```python
from build123d import *

# Parameters (mm, degrees)
BOSS_EXTRUDE1_DEPTH = 6.35
FILLET1_R           = 3.302
FILLET2_R           = 3.302


with BuildPart() as part:
    # Sketch1 → Boss-Extrude1 (new body)
    with BuildSketch(Plane.XY):
        with BuildLine():
            Line((-43.182028134, 76.689298909), (-24.787442952, -5.544607461))
            ThreePointArc((-24.787442952, -5.544607461), (0, -25.4), (24.787442952, -5.544607461))
            Line((24.787442952, -5.544607461), (43.182028134, 76.689298909))
            ThreePointArc((43.182028134, 76.689298909), (0, 88.011), (-43.182028134, 76.689298909))
        make_face()
        with BuildLine():
            Line((-6.704060429, 15.0876), (6.704060429, 15.0876))
            ThreePointArc((6.704060429, 15.0876), (11.674332957, 11.674332957), (15.0876, 6.704060429))
            Line((15.0876, 6.704060429), (15.0876, -6.704060429))
            ThreePointArc((15.0876, -6.704060429), (11.674332957, -11.674332957), (6.704060429, -15.0876))
            Line((6.704060429, -15.0876), (-6.704060429, -15.0876))
            ThreePointArc((-6.704060429, -15.0876), (-11.674332957, -11.674332957), (-15.0876, -6.704060429))
            Line((-15.0876, -6.704060429), (-15.0876, 6.704060429))
            ThreePointArc((-15.0876, 6.704060429), (-11.674332957, 11.674332957), (-6.704060429, 15.0876))
        make_face(mode=Mode.SUBTRACT)
        with BuildLine():
            ThreePointArc((-34.124988821, 73.18127185), (0, 80.7466), (34.124988821, 73.18127185))
            ThreePointArc((34.124988821, 73.18127185), (35.218416261, 70.177102101), (32.214247077, 69.083673111))
            ThreePointArc((32.214247077, 69.083673111), (0, 76.2254), (-32.214247077, 69.083673111))
            ThreePointArc((-32.214247077, 69.083673111), (-35.218416261, 70.177102101), (-34.124988821, 73.18127185))
        make_face(mode=Mode.SUBTRACT)
    extrude(amount=BOSS_EXTRUDE1_DEPTH)

    # Fillet1
    fillet1_edges = [part.edges().sort_by_distance(p)[0] for p in [
        (-15.0876, 6.704060429, 3.175),
        (-15.0876, -6.704060429, 3.175),
        (-6.704060429, -15.0876, 3.175),
        (6.704060429, -15.0876, 3.175),
        (15.0876, -6.704060429, 3.175),
        (15.0876, 6.704060429, 3.175),
        (6.704060429, 15.0876, 3.175),
        (-6.704060429, 15.0876, 3.175),
    ]]
    fillet(fillet1_edges, radius=FILLET1_R)

    # Fillet2
    fillet2_edges = [part.edges().sort_by_distance(p)[0] for p in [
        (43.182028134, 76.689298909, 3.175),
        (-43.182028134, 76.689298909, 3.175),
    ]]
    fillet(fillet2_edges, radius=FILLET2_R)


solid = part.part
```
Model file for the job. Use its own axes, mm. A direction names the side the tool comes from. Coordinates: 2 decimals unless noted, no trailing zeros. Write each loop counter-clockwise with the first axis right and the second up, starting at its lowest first coordinate (ties: lowest second). Pieces come first, ordered by that corner, then holes. Notation, with made-up numbers: (-23, 14) - (-3, 14) arc R16 cw to (-3, 42) - close; hole circle Ø10 at (15, 73.25). An arc over 180 degrees is marked (long way). Use a Markdown table: item, result. Add a question column.
Item 1: Drop flat-ended pins along their axis: pin 1 (1.5 mm diameter, centred on y = -4.5, z = 1.5, fed in from -X); pin 2 (1 mm diameter, centred on x = -18, z = 5, fed in from +Y); pin 3 (1.5 mm diameter, centred on y = 43.5, z = 5, fed in from -X); pin 4 (12 mm diameter, centred on x = -32.5, y = 45, fed in from -Z). Give the stop position or say it passes through.
Item 2: Band-saw the part on B-B, the plane y = 79.5. Write the cut outline in (x, z), and give its area (3 significant figures).
Item 3: 3-axis set-ups, long thin cutter, end or side, ignore diameter. For faces 1 (the face through (-11.73, 11.62, 3.13)), 2 (the face through (-1, 45, 0)): which of +Z, -Z, +X, -X, +Y, -Y reach the whole face in a straight line?
Item 4: Drill centre lines: line 1 along Y through (x, z) = (0.5, 4.25); line 2 along Y through (x, z) = (3.5, 3.5) (3 decimals); line 3 along Y through (x, z) = (16.5, 1.5). Where is each one in solid material? Low to high.
Item 5: Band-saw the part on D-D, the plane y = -1.5. Write the cut outline in (x, z).
Item 6: Band-saw the part on A-A, the plane z = 3.5. Write the cut outline in (x, y).
Item 7: Two-plate mould, pull along X, no slides. Class faces 3 (the face through (42.4, 76.39, 3.22)), 4 (the face through (-42.425, 76.339, 3.219)), 5 (the face through (0, -15.088, 3)), 6 (the face through (0.6, 88.01, 3.13)): pulls with the +X half, pulls with the -X half, needs draft (parallel to the pull), parting line crosses it, or undercut.
Item 8: Band-saw the part on C-C, the plane x = -4. Write the cut outline in (y, z), and give its area (3 significant figures).
A:
| question | item | result |
|---|---|---|
| 1 | pin 1 | stops at x = -25.19 |
| 1 | pin 2 | stops at y = 86.25 |
| 1 | pin 3 | stops at x = -35.93 |
| 1 | pin 4 | stops at z = 0 |
| 2 | outline | (-37.76, 0) - (-14.13, 0) - (-14.13, 6.35) - (-37.76, 6.35) - close; (14.13, 0) - (37.76, 0) - (37.76, 6.35) - (14.13, 6.35) - close |
| 2 | area | 300 mm² |
| 3 | face 1 | +Z, -Z |
| 3 | face 2 | -Z, +X, -X, +Y, -Y |
| 4 | line 1 | y = -25.4 to -15.09, 15.09 to 76.22, 80.75 to 88.01 |
| 4 | line 2 | y = -25.158 to -15.088, 15.088 to 76.145, 80.671 to 87.941 |
| 4 | line 3 | y = -19.31 to 74.42, 79.04 to 86.45 |
| 5 | outline | (-25.69, 0) - (-15.09, 0) - (-15.09, 6.35) - (-25.69, 6.35) - close; (15.09, 0) - (25.69, 0) - (25.69, 6.35) - (15.09, 6.35) - close |
| 6 | outline | (-42.64, 74.26) - (-24.79, -5.54) arc R25.4 ccw to (24.79, -5.54) - (42.64, 74.26) arc R3.3 ccw to (40.95, 77.9) arc R88.01 ccw to (-40.95, 77.9) arc R3.3 ccw to start; hole (-34.12, 73.18) arc R2.26 ccw to (-32.21, 69.08) arc R76.23 cw to (32.21, 69.08) arc R2.26 ccw to (34.12, 73.18) arc R80.75 ccw to start; hole (-15.09, -5.96) arc R3.3 ccw to (-14.73, -7.45) arc R16.51 ccw to (-7.45, -14.73) arc R3.3 ccw to (-5.96, -15.09) - (5.96, -15.09) arc R3.3 ccw to (7.45, -14.73) arc R16.51 ccw to (14.73, -7.45) arc R3.3 ccw to (15.09, -5.96) - (15.09, 5.96) arc R3.3 ccw to (14.73, 7.45) arc R16.51 ccw to (7.45, 14.73) arc R3.3 ccw to (5.96, 15.09) - (-5.96, 15.09) arc R3.3 ccw to (-7.45, 14.73) arc R16.51 ccw to (-14.73, 7.45) arc R3.3 ccw to (-15.09, 5.96) - close |
| 7 | face 3 | pulls with the +X half |
| 7 | face 4 | pulls with the -X half |
| 7 | face 5 | undercut |
| 7 | face 6 | parting line crosses it |
| 8 | outline | (-25.08, 0) - (-15.09, 0) - (-15.09, 6.35) - (-25.08, 6.35) - close; (15.09, 0) - (76.12, 0) - (76.12, 6.35) - (15.09, 6.35) - close; (80.65, 0) - (87.92, 0) - (87.92, 6.35) - (80.65, 6.35) - close |
| 8 | area | 497 mm² |
